```python
from build123d import *

# Parameters (mm, degrees)
SKETCH_1_R               = 11
EXTRUDE_1_DEPTH          = 6
EXTRUDE_2_DEPTH          = 25
PATTERN_CIRCULAR_1_COUNT = 7
SKETCH_4_R               = 35
SKETCH_4_R_2             = 18
CUT_EXTRUDE_2_DEPTH      = 25
FILLET_1_R               = 0.5
SKETCH_2_R               = 4.1
CUT_EXTRUDE_1_DEPTH      = 5


with BuildPart() as part:
    # Эскиз1 → Бобышка-Вытянуть1 (new body)
    with BuildSketch(Plane(origin=(0, 0, 0), x_dir=(1, 0, 0), z_dir=(0, 1, 0))):
        with Locations(Location((0, 0, 0), (0, 0, 270))):
            Circle(SKETCH_1_R)
    extrude(amount=EXTRUDE_1_DEPTH)

    # Эскиз3 → Бобышка-Вытянуть2 (add)
    with BuildSketch(Plane.XY):
        with BuildLine():
            Line((-3.7, 1.34), (-3.7, 1))
            add(Edge.make_bspline(
                [(3.8, 4.78), (0.931582196, 4.533244366), (-1.689682262, 2.992121942), (-3.7, 1)],
                knots=[0, 0, 0, 0, 1, 1, 1, 1], degree=3))
            Line((3.8, 4.78), (3.8, 5.12))
            add(Edge.make_bspline(
                [(3.8, 5.12), (0.931582196, 4.873244366), (-1.689682262, 3.332121942), (-3.7, 1.34)],
                knots=[0, 0, 0, 0, 1, 1, 1, 1], degree=3))
        make_face()
    extrude_2 = extrude(amount=EXTRUDE_2_DEPTH)

    # Круговой массив1: Бобышка-Вытянуть2 ×7 about axis
    pattern_circular_1_axis = Axis((0, 6, 0), (0, 1, 0))
    for i in range(1, PATTERN_CIRCULAR_1_COUNT):
        add(extrude_2.rotate(pattern_circular_1_axis, i * 360 / PATTERN_CIRCULAR_1_COUNT))

    # Эскиз4 → Вырез-Вытянуть2 (cut)
    with BuildSketch(Plane(origin=(0, 6, 0), x_dir=(1, 0, 0), z_dir=(0, 1, 0))):
        Circle(SKETCH_4_R)
        Circle(SKETCH_4_R_2, mode=Mode.SUBTRACT)
    extrude(amount=-CUT_EXTRUDE_2_DEPTH, mode=Mode.SUBTRACT)

    # Скругление1
    fillet_1_edges = [part.edges().sort_by_distance(p)[0] for p in [
        (0, 6, -11),
    ]]
    fillet(fillet_1_edges, radius=FILLET_1_R)

    # Эскиз2 → Вырез-Вытянуть1 (cut)
    with BuildSketch(Plane.XZ):
        with Locations(Location((0, 0, 0), (0, 0, 270))):
            Circle(SKETCH_2_R)
    extrude(amount=-CUT_EXTRUDE_1_DEPTH, mode=Mode.SUBTRACT)


solid = part.part
```
Build history of the part. All positions in model axes, mm. A direction names the side the tool comes from. Round coordinates to 2 decimals unless told otherwise and drop trailing zeros. Loops run counter-clockwise (first coordinate to the right, second up) from the corner with the lowest first, then second, coordinate; pieces in that order, holes last.
Item 1: Which spindle directions (+Z, -Z, +X, -X, +Y, -Y) get a long thin tool onto all of the face, cutting with end or side? Do faces 4 (the face through (9.275, 2.712, 5.914)), 5 (the face through (-9.458, 4.948, -10.882)), 6 (the face through (12.71, 4.95, -6.8)). Say none if no direction does.
Item 2: Saw through at A-A (y = 0.5). List the corners of the cut face in (x, z).
Item 3: Two-plate mould, pull along X, no slides. Class faces 1 (the face through (-14.4, 4.95, 0.61)), 2 (the face through (4.065, 2.465, 0.534)), 3 (the face through (0, 6, 0)): released by +X, released by -X, zero draft, split by the parting line, or undercut.
Item 4: Pin check, flat tips, straight feed: P1, Ø1, axis at x = -12, z = -1.5, coming from the -Y side; P2, Ø3, axis at y = 2.5, z = 11.5, coming from the +X side; P3, Ø4, axis at x = 1.5, z = -1, coming from the -Y side. Stop position of each tip, or through.
Item 5: Drill centre lines: line 1 along X through (y, z) = (3.7, 0); line 2 along X through (y, z) = (3, 9.5); line 3 along X through (y, z) = (2.25, 5.5). Where is each one in solid material? Low to high.
Worked answers:
1. face 4: none
1. face 5: -X, +Y, -Y
1. face 6: -Z, +Y, -Y
2. outline: circle Ø22 at (0, 0); hole circle Ø8.2 at (0, 0)
3. face 1: released by -X
3. face 2: undercut
3. face 3: zero draft
4. P1: stops at y = 4.01
4. P2: stops at x = 14.32
4. P3: stops at y = 5
5. line 1: x = -11 to -4.1, 4.1 to 11
5. line 2: x = -14.67 to -13.85, -5.55 to 5.55, 9.16 to 9.97
5. line 3: x = -11.23 to -10.55, -9.53 to 9.53
